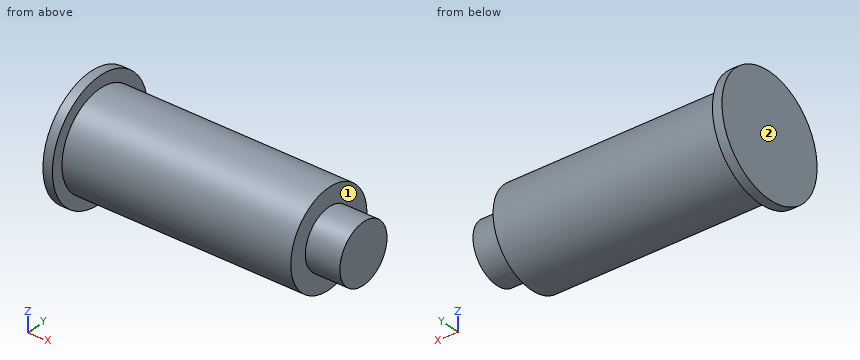
from build123d import *

# Parameters (mm, degrees)
F2_R     = 12.375
F3_DEPTH = 14.5


with BuildPart() as f1:
    # F0 (on Front) → F1 (revolve)
    with BuildSketch(Plane.XZ):
        Polygon((-100, 0), (0, 0), (0, 20), (-96, 20), (-96, 25), (-100, 25), (-100, 20), align=None)
    revolve(axis=Axis((-50, 0, 0), (-1, 0, 0)))

    # F2 (on face) → F3 (join)
    with BuildSketch(Plane.YZ):
        Circle(F2_R)
    extrude(amount=F3_DEPTH)


solid = f1.part
The model under review builds one solid part; all positions refer to its coordinate system, in mm. Face numbers are marked on the shaded views. A direction names the side the tool comes from. Round coordinates to 2 decimals unless told otherwise and drop trailing zeros. Write each loop counter-clockwise with the first axis right and the second up, starting at its lowest first coordinate (ties: lowest second). Pieces come first, ordered by that corner, then holes. Notation, with made-up numbers: M 59,-23.75 L 91,-23.75 A21 ccw 91,14.25 Z; hole C -36,-35 d9. An arc over 180 degrees is marked long. Answer as CSV lines item,"result". Start each with the question number.
Q1. Clearance check with flat-ended pins moving along their axes: P1, Ø1.5, axis at x = -42.5, z = 15, coming from the -Y side; P2, Ø5, axis at x = -26, z = -9, coming from the -Y side; P3, Ø3, axis at x = -74.5, z = 2.5, coming from the +Y side (3 decimals). State where each tip first meets the part, or that it passes through.
Q2. Tool access review of the marked faces 1 and 2: name each direction out of +Z, -Z, +X, -X, +Y, -Y from which nothing blocks a thin tool from reaching the whole face with its end or side.
Q3. Consider section A-A, the plane z = 0. Give the boundary of the cut face in (x, y) (3 decimals).
Q4. Consider section C-C, the plane x = -79.5. Give the boundary of the cut face in (y, z), then the cut area to 3 significant figures.
Q5. Wall thickness on line 1 along X through (y, z) = (-16, 1.5); line 2 along X through (y, z) = (-19, -12.5); line 3 along Y through (x, z) = (-32, 3.5): over which ranges is each line inside the solid? List them lowest first.
Q6. Consider section D-D, the plane z = 18.5. Give the boundary of the cut face in (x, y).
Result set:
1,P1,"stops at y = -14.03"
1,P2,"stops at y = -18.91"
1,P3,"stops at y = 19.975"
2,face 1,"+X"
2,face 2,"+Z, -Z, -X, +Y, -Y"
3,outline,"M -100,-25 L -96,-25 L -96,-20 L 0,-20 L 0,-12.375 L 14.5,-12.375 L 14.5,12.375 L 0,12.375 L 0,20 L -96,20 L -96,25 L -100,25 Z"
4,outline,"C 0,0 d40"
4,area,"1,260 mm²"
5,line 1,"x = -100 to 0"
5,line 2,"x = -100 to -96"
5,line 3,"y = -19.69 to 19.69"
6,outline,"M -100,-16.82 L -96,-16.82 L -96,-7.6 L 0,-7.6 L 0,7.6 L -96,7.6 L -96,16.82 L -100,16.82 Z"
